```python
from build123d import *

# Parameters (mm, degrees)
HEAD_BOSS_EXTRUDE1_OUTLINE_R = 3.5
HEAD_BOSS_EXTRUDE1_DEPTH     = 3.5
HEAD_HEX_CUT_EXTRUDE1_DEPTH  = 2.8
SKETCH2_R                    = 1.5
SCREW_BOSS_EXTRUDE2_DEPTH    = 55


# Read off the part's stored shape, not the designer's step: Head Boss-Extrude1
with BuildPart() as part:
    # Head Boss-Extrude1 outline → Head Boss-Extrude1 (new body)
    with BuildSketch(Plane.XY):
        Circle(HEAD_BOSS_EXTRUDE1_OUTLINE_R)
    extrude(amount=HEAD_BOSS_EXTRUDE1_DEPTH)

    # Sketch3 → Head Hex Cut-Extrude1 (cut)
    with BuildSketch(Plane.XY.offset(3.5)):
        Polygon((-1.010362971, 1.75), (1.010362971, 1.75), (2.020725942, 0), (1.010362971, -1.75), (-1.010362971, -1.75), (-2.020725942, 0), align=None)
    extrude(amount=-HEAD_HEX_CUT_EXTRUDE1_DEPTH, mode=Mode.SUBTRACT)

    # Sketch2 → Screw Boss-Extrude2 (add)
    with BuildSketch(Plane.XY):
        Circle(SKETCH2_R)
    extrude(amount=-SCREW_BOSS_EXTRUDE2_DEPTH)


solid = part.part
```
Part model, mm, in its own coordinate system. A direction names the side the tool comes from. Round coordinates to 2 decimals unless told otherwise and drop trailing zeros. Write each loop counter-clockwise with the first axis right and the second up, starting at its lowest first coordinate (ties: lowest second). Pieces come first, ordered by that corner, then holes.
Item 1: Cut at B-B, the plane y = 0.75. Give the cut face in (x, z).
Results:
outline: (-3.42, 0) - (-1.3, 0) - (-1.3, -55) - (1.3, -55) - (1.3, 0) - (3.42, 0) - (3.42, 3.5) - (1.59, 3.5) - (1.59, 0.7) - (-1.59, 0.7) - (-1.59, 3.5) - (-3.42, 3.5) - close
Item 2: Cut at C-C, the plane z = -38.5. Give the cut face in (x, y).
Results:
outline: circle Ø3 at (0, 0)
Item 3: Cut at A-A, the plane x = 0. Give the cut face in (y, z).
Results:
outline: (-3.5, 0) - (-1.5, 0) - (-1.5, -55) - (1.5, -55) - (1.5, 0) - (3.5, 0) - (3.5, 3.5) - (1.75, 3.5) - (1.75, 0.7) - (-1.75, 0.7) - (-1.75, 3.5) - (-3.5, 3.5) - close
Item 4: Cut at D-D, the plane x = -2.5. Give the cut face in (y, z).
Results:
outline: (-2.45, 0) - (2.45, 0) - (2.45, 3.5) - (-2.45, 3.5) - close
Item 5: Probe L1, parallel to Z at x = -1, y = -0.25; L2, parallel to Z at x = -1.5, y = -1; L3, parallel to X at y = -0.5, z = -8.5. List the from-to ranges inside material, lowest first.
Results:
L1: z = -55 to 0.7
L2: z = 0 to 3.5
L3: x = -1.41 to 1.41
Item 6: Which spindle directions (+Z, -Z, +X, -X, +Y, -Y) get a long thin tool onto all of the face, cutting with end or side? Do faces 1 (the cylindrical face through (-1.5, 0.07, -27.12)), 2 (the flat face through (-2, -1, 3.5)), 3 (the flat face through (1.5, -0.9, 2.1)). Say none if no direction does.
Results:
face 1: -Z
face 2: +Z, +X, -X, +Y, -Y
face 3: +Z
Item 7: Two-plate mould, pull along Y, no slides. Class faces 4 (the flat face through (0, 1.75, 2)), 5 (the cylindrical face through (3.233, -1.341, 1.726)), 6 (the flat face through (0, 0, -55)): +Y half, -Y half, draft (parallel to the pull), parting line (faces both ways), or undercut.
Results:
face 4: undercut
face 5: parting line
face 6: draft
Item 8: Drop a flat-ended pin along its axis: pin 1 Ø1 at (x, y) = (-0.5, 0) entering from +Z. Give the stop position or say it passes through.
Results:
pin 1: stops at z = 0.7
